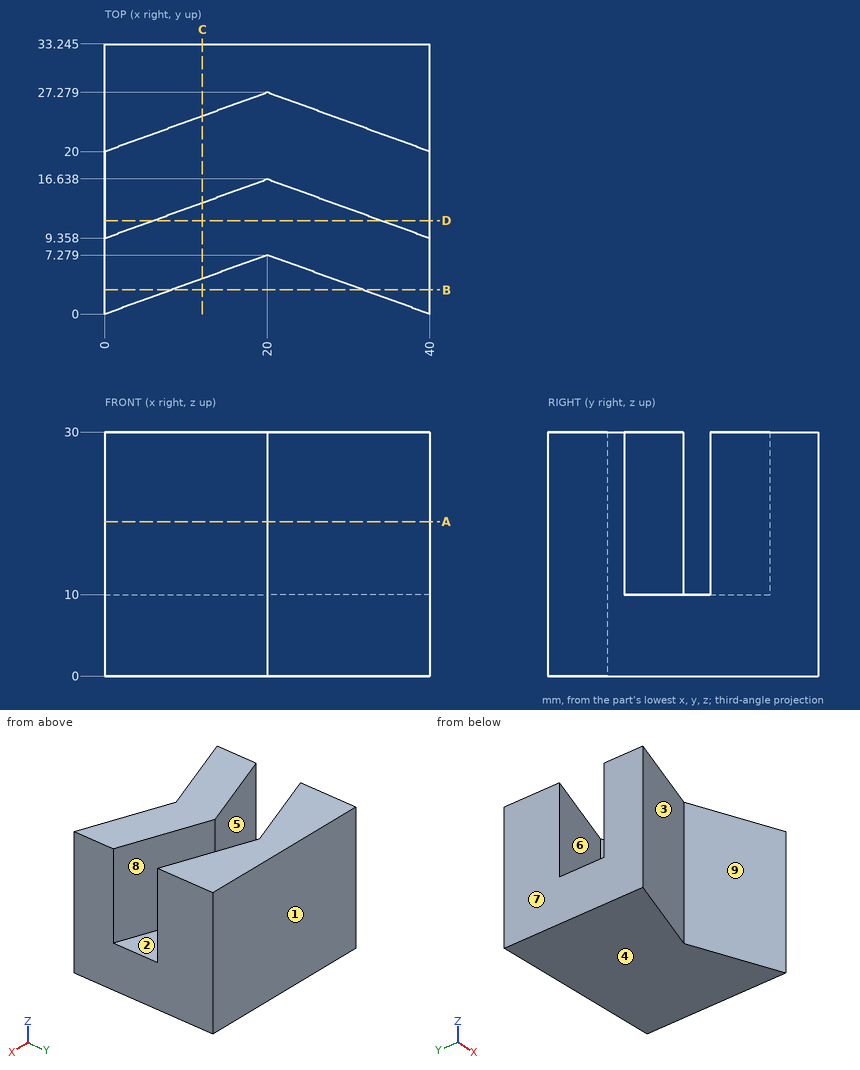
Design review of the part shown in the three views and the two pictorial views. Dimensions are in mm from the part's minimum x, y and z. A direction names the side the tool comes from. Give positions to 0.01 mm unless a question says otherwise; leave off trailing zeros. Loops run counter-clockwise (first coordinate to the right, second up) from the corner with the lowest first, then second, coordinate; pieces in that order, holes last. Notation, with made-up numbers: (-32, 57) -> (14, 57) arc R8 ccw to (14, 63) -> close; hole circle Ø3 at (77.5, 36.5). An arc over 180 degrees is marked (long way). Answer as a JSON object with one key per item and string values. Group by question number.
Q1. Tool access review of the marked faces 5, 6, 7, 8 and 9: name each direction out of +Z, -Z, +X, -X, +Y, -Y from which nothing blocks a thin tool from reaching the whole face with its end or side.
Q2. Take a section at A-A (z = 19). Write out the cut boundary in (x, y) (1 decimal).
Q3. Draft analysis for pull direction Y (two halves, no side actions). For the marked faces 1, 2, 3 and 4, state which applies: pulls with the +Y half, pulls with the -Y half, needs draft (parallel to the pull), parting line crosses it, or undercut.
Q4. Take a section at D-D (y = 11.5). Write out the cut boundary in (x, z) (1 decimal), plus the area to 3 significant figures.
Q5. Take a section at C-C (x = 12). Write out the cut boundary in (y, z) (1 decimal).
Q6. Insertion check: pin 1 (1.5 mm diameter, centred on y = 3.5, z = 3, fed in from -X); pin 2 (2 mm diameter, centred on x = 13.5, y = 21.5, fed in from +Z); pin 3 (4 mm diameter, centred on x = 33, z = 14, fed in from -Y). Each pin has a flat end and moves straight along its axis. Give the tip position at first contact, or say it passes through.
Q7. Wall thickness on line 1 along Z through (x, y) = (7, 12); line 2 along Y through (x, z) = (18, 15) (1 decimal); line 3 along Y through (x, z) = (3.5, 13) (1 decimal): over which ranges is each line inside the solid? List them lowest first.
Q8. Take a section at B-B (y = 3). Write out the cut boundary in (x, z).
Answer below:
{
 "1": {"face 5": "+Z, -X", "face 6": "+Z", "face 7": "+Z, -Z, -X, +Y, -Y", "face 8": "+Z, +X", "face 9": "+Z, -Z, -Y"},
 "2": {"outline": "(0, 0) -> (20, 7.3) -> (40, 0) -> (40, 9.4) -> (20, 16.6) -> (0, 9.4) -> close; (0, 20) -> (20, 27.3) -> (40, 20) -> (40, 33.2) -> (0, 33.2) -> close"},
 "3": {"face 1": "pulls with the +Y half", "face 2": "undercut", "face 3": "pulls with the -Y half", "face 4": "needs draft"},
 "4": {"outline": "(0, 0) -> (40, 0) -> (40, 10) -> (34.1, 10) -> (34.1, 30) -> (5.9, 30) -> (5.9, 10) -> (0, 10) -> close", "area": "965 mm2"},
 "5": {"outline": "(4.4, 0) -> (33.2, 0) -> (33.2, 30) -> (24.4, 30) -> (24.4, 10) -> (13.7, 10) -> (13.7, 30) -> (4.4, 30) -> close"},
 "6": {"pin 1": "stops at x = 0", "pin 2": "stops at z = 10", "pin 3": "stops at y = 1.82"},
 "7": {"line 1": "z = 0 to 10", "line 2": "y = 6.6 to 15.9, 26.6 to 33.2", "line 3": "y = 1.3 to 10.6, 21.3 to 33.2"},
 "8": {"outline": "(0, 0) -> (8.24, 0) -> (8.24, 30) -> (0, 30) -> close; (31.76, 0) -> (40, 0) -> (40, 30) -> (31.76, 30) -> close"}
}
